Design review of the part built by this model. Coordinates are the model's own, in mm. Give positions to 0.01 mm unless a question says otherwise; leave off trailing zeros. Write each loop counter-clockwise with the first axis right and the second up, starting at its lowest first coordinate (ties: lowest second). Pieces come first, ordered by that corner, then holes. Notation, with made-up numbers: (-35.5, -40) - (-22.5, -40) arc R24 ccw to (-22.5, -9) - close; hole circle Ø3 at (0, 2.5). An arc over 180 degrees is marked (long way). Use a Markdown table: item, result. Add a question column.
```python
from build123d import *

# Parameters (mm, degrees)
SKETCH1_R                          = 4.7625
BOSS_EXTRUDE1_DEPTH                = 6.35
TAP_DRILL_FOR_6_32_TAP2_AT_2_COUNT = 2
TAP_DRILL_FOR_6_32_TAP2_AT_2_PITCH = 14.2875
SKETCH18_W                         = 63.246
SKETCH18_H                         = 14.2875
CUT_EXTRUDE1_DEPTH                 = 148.950291114
FILLET1_R                          = 2.54
TAP_DRILL_FOR_6_32_TAP4_D          = 2.7051
TAP_DRILL_FOR_6_32_TAP1_AT_2_COUNT = 2
TAP_DRILL_FOR_6_32_TAP1_AT_2_PITCH = 28.085742046
TAP_DRILL_FOR_6_32_TAP1_AT_3_COUNT = 2
TAP_DRILL_FOR_6_32_TAP1_AT_3_PITCH = 24.165817496
SKETCH23_W                         = 6.35
SKETCH23_H                         = 8.001
CUT_EXTRUDE2_DEPTH                 = 3.175


with BuildPart() as part:
    # Sketch1 → Boss-Extrude1 (new body)
    with BuildSketch(Plane(origin=(0, 0, 0), x_dir=(0, 0, -1), z_dir=(1, 0, 0))):
        Polygon((0, 0), (-17.414327494, 30.1625), (-55.0164, 30.1625), (-55.0164, 26.9875), (-89.6874, 26.9875), (-89.6874, 30.1625), (-127.289472506, 30.1625), (-144.7038, 0), (-86.8299, 0), (-86.8299, 1.5875), (-57.8739, 1.5875), (-57.8739, 0), align=None)
        with Locations((-111.9124, 14.2875)):
            Circle(SKETCH1_R, mode=Mode.SUBTRACT)
        with Locations((-32.7914, 14.2875)):
            Circle(SKETCH1_R, mode=Mode.SUBTRACT)
    extrude(amount=BOSS_EXTRUDE1_DEPTH)

    # Sketch14 → Tap Drill for #6-32 Tap2 (revolve, cut)
    with BuildSketch(Plane(origin=(3.175, 8.165454744, 139.989472506), x_dir=(0, -0.8660254037844365, 0.500000000000004), z_dir=(1, 0, 0))):
        Polygon((0, 0), (0, 7.16269403), (1.35255, 6.35), (1.35255, 0), align=None)
    tap_drill_for_6_32_tap2 = revolve(axis=Axis((3.175, 11.340454744, 145.48873382), (0, -0.5000000000000039, -0.8660254037844364)), mode=Mode.SUBTRACT)

    # Tap Drill for #6-32 Tap2 at 2: Tap Drill for #6-32 Tap2 ×2
    with Locations(*[Vector(0, 0.8660254037844364, -0.500000000000004) * (i * TAP_DRILL_FOR_6_32_TAP2_AT_2_PITCH) for i in range(1, TAP_DRILL_FOR_6_32_TAP2_AT_2_COUNT)]):
        add(tap_drill_for_6_32_tap2, mode=Mode.SUBTRACT)

    # Sketch18 → Cut-Extrude1 (cut, through all)
    with BuildSketch(Plane.ZY):
        Polygon((16.12265, 6.35), (25.64765, 6.35), (25.64765, 22.847783942), align=None)
        with Locations((72.3519, 15.08125)):
            Rectangle(SKETCH18_W, SKETCH18_H)
        Polygon((119.05615, 6.35), (119.05615, 22.847783942), (128.58115, 6.35), align=None)
    extrude(amount=-CUT_EXTRUDE1_DEPTH, mode=Mode.SUBTRACT)

    # Fillet1
    fillet1_edges = [part.edges().sort_by_distance(p)[0] for p in [
        (3.175, 7.9375, 40.7289),
        (3.175, 22.225, 40.7289),
        (3.175, 22.225, 103.9749),
        (3.175, 7.9375, 103.9749),
    ]]
    fillet(fillet1_edges, radius=FILLET1_R)

    # Tap Drill for #6-32 Tap4 (through all)
    with Locations(Plane(origin=(0, 26.9875, 0), x_dir=(1, 0, 0), z_dir=(0, 1, 0))):
        with Locations((3.175, -72.3519)):
            Hole(TAP_DRILL_FOR_6_32_TAP4_D / 2)

    # Mirror1: Tap Drill for #6-32 Tap2 across plane
    add(tap_drill_for_6_32_tap2.mirror(Plane(origin=(0, 0, 72.3519), x_dir=(1, 0, 0), z_dir=(0, 0, -1))), mode=Mode.SUBTRACT)

    # Mirror1 copy 1 sketch → Mirror1 copy 1 (revolve, cut)
    with BuildSketch(Plane(origin=(3.175, 20.5387927, 11.858077494), x_dir=(0, -0.8660254037844365, -0.500000000000004), z_dir=(1, 0, 0))):
        Polygon((0, 0), (0, -7.16269403), (1.35255, -6.35), (1.35255, 0), align=None)
    revolve(axis=Axis((3.175, 23.7137927, 6.35881618), (0, 0.5000000000000039, -0.8660254037844364)), mode=Mode.SUBTRACT)

    # Sketch12 → Tap Drill for #6-32 Tap1 (revolve, cut)
    with BuildSketch(Plane(origin=(6.35, 25.4, 118.2624), x_dir=(0, 0, -1), z_dir=(0, 1, 0))):
        Polygon((0, 0), (0, 7.16269403), (1.35255, 6.35), (1.35255, 0), align=None)
    tap_drill_for_6_32_tap1 = revolve(axis=Axis((12.7, 25.4, 118.2624), (-1, 0, 0)), mode=Mode.SUBTRACT)

    # Tap Drill for #6-32 Tap1 at 2: Tap Drill for #6-32 Tap1 ×2
    with Locations(*[Vector(0, -0.734803444627488, -0.6782801027330657) * (i * TAP_DRILL_FOR_6_32_TAP1_AT_2_PITCH) for i in range(1, TAP_DRILL_FOR_6_32_TAP1_AT_2_COUNT)]):
        add(tap_drill_for_6_32_tap1, mode=Mode.SUBTRACT)

    # Tap Drill for #6-32 Tap1 at 3: Tap Drill for #6-32 Tap1 ×2
    with Locations(*[Vector(0, -0.8539955250185772, 0.5202803506267027) * (i * TAP_DRILL_FOR_6_32_TAP1_AT_3_PITCH) for i in range(1, TAP_DRILL_FOR_6_32_TAP1_AT_3_COUNT)]):
        add(tap_drill_for_6_32_tap1, mode=Mode.SUBTRACT)

    # Mirror2: Tap Drill for #6-32 Tap1 across plane
    add(tap_drill_for_6_32_tap1.mirror(Plane(origin=(0, 0, 72.3519), x_dir=(1, 0, 0), z_dir=(0, 0, -1))), mode=Mode.SUBTRACT)

    # Mirror2 copy 1 sketch → Mirror2 copy 1 (revolve, cut)
    with BuildSketch(Plane(origin=(6.35, 4.7625, 45.4914), x_dir=(0, 0, 1), z_dir=(0, 1, 0))):
        Polygon((0, 0), (0, -7.16269403), (1.35255, -6.35), (1.35255, 0), align=None)
    revolve(axis=Axis((12.7, 4.7625, 45.4914), (1, 0, 0)), mode=Mode.SUBTRACT)

    # Mirror2 copy 2 sketch → Mirror2 copy 2 (revolve, cut)
    with BuildSketch(Plane(origin=(6.35, 4.7625, 13.8684), x_dir=(0, 0, 1), z_dir=(0, 1, 0))):
        Polygon((0, 0), (0, -7.16269403), (1.35255, -6.35), (1.35255, 0), align=None)
    revolve(axis=Axis((12.7, 4.7625, 13.8684), (1, 0, 0)), mode=Mode.SUBTRACT)

    # Sketch23 → Cut-Extrude2 (cut)
    with BuildSketch(Plane(origin=(0, 0, 0), x_dir=(-1, 0, 0), z_dir=(0, 0.49999999999999806, -0.8660254037844397))):
        with Locations((-3.175, 23.460115329)):
            Rectangle(SKETCH23_W, SKETCH23_H)
        with Locations((-3.175, 9.058315329)):
            Rectangle(SKETCH23_W, SKETCH23_H)
    cut_extrude2 = extrude(amount=-CUT_EXTRUDE2_DEPTH, mode=Mode.SUBTRACT)

    # Mirror3: Cut-Extrude2 across plane
    add(cut_extrude2.mirror(Plane(origin=(0, 0, 72.3519), x_dir=(1, 0, 0), z_dir=(0, 0, -1))), mode=Mode.SUBTRACT)


solid = part.part
```
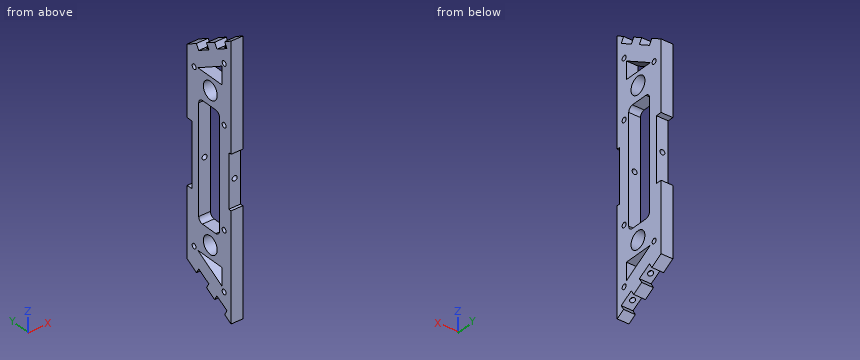
(1) Add section A-A (y = 25.4). State the section outline as (x, z) points (3 decimals), and give its area (3 significant figures).
(2) Add section C-C (y = 12.5). State the section outline as (x, z) points, and give its area (3 significant figures).
(3) Add section B-B (z = 42). State the section outline as (x, y) points, and give its area (3 significant figures).
(4) For line 1 along Z through (x, y) = (3.5, 25.5); line 2 along Z through (x, y) = (3.75, 18); line 3 along Z through (x, y) = (2, 20.5), list the stretches that pass through material, from the lowest coordinate up.
(5) Insertion check: pin 1 (1 mm diameter, centred on x = 3, y = 28.5, fed in from +Z); pin 2 (1 mm diameter, centred on y = 20.5, z = 49, fed in from +X); pin 3 (3 mm diameter, centred on y = 4.76, z = 99.21, fed in from +X); pin 4 (3 mm diameter, centred on x = 3, z = 66.5, fed in from +Y). Each pin has a flat end and moves straight along its axis. Give the tip position at first contact, or say it passes through.
Answers follow:
| question | item | result |
|---|---|---|
| 1 | outline | (0, 14.665) - (6.35, 14.665) - (6.35, 25.089) - (0, 25.089) - close; (0, 27.794) - (6.35, 27.794) - (6.35, 116.91) - (0, 116.91) - close; (0, 119.615) - (6.35, 119.615) - (6.35, 130.039) - (0, 130.039) - close; hole circle Ø2.705 at (3.175, 72.352) |
| 1 | area | 693 mm^2 |
| 2 | outline | (0, 7.22) - (6.35, 7.22) - (6.35, 19.67) - (0, 19.67) - close; (0, 25.65) - (6.35, 25.65) - (6.35, 28.38) - (0, 28.38) - close; (0, 37.21) - (6.35, 37.21) - (6.35, 40.73) - (0, 40.73) - close; (0, 103.97) - (6.35, 103.97) - (6.35, 107.5) - (0, 107.5) - close; (0, 116.33) - (6.35, 116.33) - (6.35, 119.06) - (0, 119.06) - close; (0, 125.03) - (6.35, 125.03) - (6.35, 137.49) - (0, 137.49) - close |
| 2 | area | 238 mm^2 |
| 3 | outline | (0, 0) - (6.35, 0) - (6.35, 8.28) - (0, 8.28) - close; (0, 21.89) - (6.35, 21.89) - (6.35, 30.16) - (0, 30.16) - close |
| 3 | area | 105 mm^2 |
| 4 | line 1 | 14.72 to 25.09, 27.79 to 71.04, 73.66 to 116.91, 119.61 to 129.98 |
| 4 | line 2 | 17.95 to 22.85, 25.65 to 29.81, 35.77 to 40.73, 103.97 to 108.93, 114.9 to 119.06, 121.86 to 126.75 |
| 4 | line 3 | 15.5 to 24.29, 25.65 to 40.86, 103.84 to 119.06, 120.41 to 129.2 |
| 5 | pin 1 | z = 128.54 |
| 5 | pin 2 | through |
| 5 | pin 3 | x = 6.35 |
| 5 | pin 4 | y = 26.99 |
